```python
from build123d import *

# Parameters (mm, degrees)
SKETCH1_R           = 3.2639
SKETCH1_R_2         = 7.9375
SKETCH1_R_3         = 4.191
BOSS_EXTRUDE4_DEPTH = 3.175
FILLET1_START       = -3.175
FILLET1_DEPTH       = 3.175


with BuildPart() as part:
    # Sketch1 → Boss-Extrude4 (new body)
    with BuildSketch(Plane(origin=(0, 0, 0), x_dir=(1, 0, 0), z_dir=(0, 1, 0))):
        with BuildLine():
            ThreePointArc((133.726592386, 29.98785526), (132.627611185, 40.61059676), (122.521356715, 44.06226552))
            Line((122.521356715, 44.06226552), (46.442862481, 25.430137021))
            ThreePointArc((46.442862481, 25.430137021), (36.958837973, 28.991331503), (30.193743977, 21.450619984))
            Line((30.193743977, 21.450619984), (-3.247611444, 13.260609947))
            ThreePointArc((-3.247611444, 13.260609947), (-13.651169136, -0.190623903), (-2.876077052, -13.346120674))
            Line((-2.876077052, -13.346120674), (23.107180797, -18.945489468))
            ThreePointArc((23.107180797, -18.945489468), (24.589406384, -19.137653713), (26.082973185, -19.081279984))
            Line((26.082973185, -19.081279984), (109.669270086, -8.913192671))
            ThreePointArc((109.669270086, -8.913192671), (113.749462268, -7.344996575), (116.60566957, -4.036025875))
            Line((116.60566957, -4.036025875), (133.726592386, 29.98785526))
        make_face()
        with Locations(Location((24.998703099, -10.168087313, 0), (0, 0, 270))):
            Circle(SKETCH1_R, mode=Mode.SUBTRACT)
        with Locations(Location((0, 0, 0), (0, 0, 270))):
            Circle(SKETCH1_R_2, mode=Mode.SUBTRACT)
        with BuildLine():
            Line((38.450716367, 11.314391845), (41.984168993, -4.864970405))
            Line((41.984168993, -4.864970405), (32.525550861, -5.272455792))
            ThreePointArc((32.525550861, -5.272455792), (24.612242842, -1.197507974), (17.07870805, -5.937919038))
            Line((17.07870805, -5.937919038), (12.189591197, -6.148546389))
            ThreePointArc((12.189591197, -6.148546389), (13.515826194, 1.926966151), (9.985636063, 9.310092839))
            Line((9.985636063, 9.310092839), (32.042893317, 14.712061629))
            ThreePointArc((32.042893317, 14.712061629), (34.888474765, 12.337435423), (38.450716367, 11.314391845))
        make_face(mode=Mode.SUBTRACT)
        with Locations(Location((39.094708942, 20.270167566, 0), (0, 0, 270))):
            Circle(SKETCH1_R, mode=Mode.SUBTRACT)
        with BuildLine():
            Line((54.876229285, -4.309569382), (78.030840873, 27.282347644))
            Line((78.030840873, 27.282347644), (100.723144875, 4.337266328))
            ThreePointArc((100.723144875, 4.337266328), (99.66914772, 1.062178575), (99.924218758, -2.368863331))
            Line((99.924218758, -2.368863331), (54.876229285, -4.309569382))
        make_face(mode=Mode.SUBTRACT)
        with BuildLine():
            Line((104.335087932, 7.90941797), (84.823475635, 27.638376771))
            Line((84.823475635, 27.638376771), (114.98908268, 35.026134276))
            ThreePointArc((114.98908268, 35.026134276), (117.570132445, 27.752761279), (124.58688197, 24.538885311))
            Line((124.58688197, 24.538885311), (115.260501822, 6.004858086))
            ThreePointArc((115.260501822, 6.004858086), (110.126982004, 8.845503757), (104.335087932, 7.90941797))
        make_face(mode=Mode.SUBTRACT)
        with Locations(Location((108.585, 0, 0), (0, 0, 270))):
            Circle(SKETCH1_R, mode=Mode.SUBTRACT)
        with BuildLine():
            Line((47.13543811, -4.64304931), (43.413738486, 12.398279038))
            ThreePointArc((43.413738486, 12.398279038), (46.36017499, 14.994407118), (47.916850432, 18.599699151))
            Line((47.916850432, 18.599699151), (69.18664036, 23.808811963))
            Line((69.18664036, 23.808811963), (48.372525925, -4.589754505))
            Line((48.372525925, -4.589754505), (47.13543811, -4.64304931))
        make_face(mode=Mode.SUBTRACT)
        with Locations(Location((124.877763158, 34.440613651, 0), (0, 0, 270))):
            Circle(SKETCH1_R_3, mode=Mode.SUBTRACT)
    extrude(amount=-BOSS_EXTRUDE4_DEPTH)

    # Fillet1: read off the stored shape, not the designer's step
    # Fillet1 outline → Fillet1 (add)
    with BuildSketch(Plane(origin=(0, 0, 0), x_dir=(1, 0, 0), z_dir=(0, 1, 0)).offset(FILLET1_START)):
        with BuildLine():
            Line((114.98908268, 35.026134276), (107.783269008, 33.261382651))
            add(Edge.make_bspline(
                [(107.783269008, 33.261382651), (113.406008329, 34.638428853), (116.240182309, 29.590764883)],
                knots=[0, 0, 0, 1, 1, 1], degree=2))
            ThreePointArc((116.240182309, 29.590764883), (115.224193881, 32.218579403), (114.98908268, 35.026134276))
        make_face()
        with BuildLine():
            Line((115.260501822, 6.004858086), (118.700286007, 12.840634961))
            add(Edge.make_bspline(
                [(118.700286007, 12.840634961), (116.082209563, 7.637812501), (110.374675184, 8.798733315)],
                knots=[0, 0, 0, 1, 1, 1], degree=2))
            ThreePointArc((110.374675184, 8.798733315), (113.042156059, 7.794511215), (115.260501822, 6.004858086))
        make_face()
        with BuildLine():
            ThreePointArc((124.58688197, 24.538885311), (121.515947768, 25.122511201), (118.779768978, 26.633994475))
            add(Edge.make_bspline(
                [(118.779768978, 26.633994475), (123.70514236, 22.786631417), (120.895795937, 17.203704037)],
                knots=[0, 0, 0, 1, 1, 1], degree=2))
            Line((120.895795937, 17.203704037), (124.58688197, 24.538885311))
        make_face()
        with BuildLine():
            ThreePointArc((9.985636063, 9.310092839), (12.154183418, 6.21824587), (13.392725611, 2.650595587))
            add(Edge.make_bspline(
                [(13.392725611, 2.650595587), (11.978146555, 9.798071891), (19.055114913, 11.531268442)],
                knots=[0, 0, 0, 1, 1, 1], degree=2))
            Line((19.055114913, 11.531268442), (9.985636063, 9.310092839))
        make_face()
        with BuildLine():
            add(Edge.make_bspline(
                [(17.07870805, -5.937919038), (13.730219916, -3.733889963), (13.649749039, 0.274057316)],
                knots=[0, 0, 0, 1, 1, 1], degree=2))
            ThreePointArc((13.649749039, 0.274057316), (13.312788421, -3.026618691), (12.189591197, -6.148546389))
            Line((12.189591197, -6.148546389), (17.07870805, -5.937919038))
        make_face()
        with BuildLine():
            ThreePointArc((99.924218758, -2.368863331), (99.607534733, 0.160507278), (100.014432232, 2.67694104))
            add(Edge.make_bspline(
                [(100.014432232, 2.67694104), (98.418154374, -2.433745878), (93.068937879, -2.664194715)],
                knots=[0, 0, 0, 1, 1, 1], degree=2))
            Line((93.068937879, -2.664194715), (99.924218758, -2.368863331))
        make_face()
    extrude(amount=FILLET1_DEPTH)


solid = part.part
```
CAD build for the part. Positions are in the model's coordinates, mm. A direction names the side the tool comes from. Coordinates: 2 decimals unless noted, no trailing zeros. Loops run counter-clockwise (first coordinate to the right, second up) from the corner with the lowest first, then second, coordinate; pieces in that order, holes last. Notation, with made-up numbers: (9, -27) - (20, -27) arc R27 cw to (20, -6) - close; hole circle Ø6 at (73, 28.25). An arc over 180 degrees is marked (long way). Return JSON: item names as keys, results as strings.
1. Band-saw the part on B-B (x = 87). Give the cut face in (y, z) (3 decimals).
Result:
{"outline": "(-3.175, -35.363) - (0, -35.363) - (0, -28.171) - (-3.175, -28.171) - close; (-3.175, -25.438) - (0, -25.438) - (0, -18.213) - (-3.175, -18.213) - close; (-3.175, 2.926) - (0, 2.926) - (0, 11.671) - (-3.175, 11.671) - close"}
2. Mould opens along X. For faces 3 (the flat face through (60, 0, -6)), 4 (the cylindrical face through (-13.652, -1.565, -0.066)), 5 (the cylindrical face through (117.345, -1.565, -28.007)) say: released by +X, released by -X, zero draft, split by the parting line, or undercut.
Result:
{"face 3": "zero draft", "face 4": "released by -X", "face 5": "undercut"}
3. Probe L1, parallel to Z at x = 25, y = -1.3; L2, parallel to Z at x = 95.5, y = -0.8; L3, parallel to X at y = -1.3, z = 0. List the from-to ranges inside material, lowest first. Write a range as from..to.
Result:
{"L1": "z = -20.18..-12.99, 1.19..6.9, 13.43..19.15", "L2": "z = -37.44..-30.25, -16.84..-9.62, 2.25..10.64", "L3": "x = -13.65..-7.94, 7.94..13.66, 40.92..46.12, 51.74..58.03, 98.68..105.32, 111.85..118.64"}
4. Band-saw the part on C-C (z = 11). Give the cut face in (x, y) (3 decimals), and give its area (3 significant figures).
Result:
{"outline": "(-8.086, -3.175) - (21.843, -3.175) - (21.843, 0) - (-8.086, 0) - close; (28.155, -3.175) - (92.515, -3.175) - (92.515, 0) - (28.155, 0) - close", "area": "299 mm2"}
5. Band-saw the part on D-D (x = 62). Give the cut face in (y, z) (3 decimals).
Result:
{"outline": "(-3.175, -29.24) - (0, -29.24) - (0, -22.049) - (-3.175, -22.049) - close; (-3.175, -14.003) - (0, -14.003) - (0, -5.41) - (-3.175, -5.41) - close; (-3.175, 4.003) - (0, 4.003) - (0, 14.712) - (-3.175, 14.712) - close"}
6. 3-axis set-ups, long thin cutter, end or side, ignore diameter. For faces 1 (the flat face through (25.46, -1.57, -13.1)), 2 (the cylindrical face through (24.568, -1.565, 19.137)): which of +Z, -Z, +X, -X, +Y, -Y reach the whole face in a straight line?
Result:
{"face 1": "+Y, -Y", "face 2": "+Z, +Y, -Y"}
7. Band-saw the part on A-A (x = 0). Give the cut face in (y, z) (1 decimal).
Result:
{"outline": "(-3.2, -14.1) - (0, -14.1) - (0, -7.9) - (-3.2, -7.9) - close; (-3.2, 7.9) - (0, 7.9) - (0, 14) - (-3.2, 14) - close"}
